```python
from build123d import *

# Parameters (mm, degrees)
F2_T     = -12.7
F3_R     = 76.2
F4_DEPTH = 781.3280539866
F6_DEPTH = 254
F7_COUNT = 24


with BuildPart() as f1:
    # F0 (on Front) → F1 (revolve)
    with BuildSketch(Plane.XZ):
        Polygon((-673.1, 0), (0, 0), (0, 781.3270539866), (-127, 781.3270539866), (-127, 400.3270539866), (-673.1, 254), align=None)
    revolve(axis=Axis((0, 0, 573.1903910637), (0, 0, 1)))

    # F2
    f2_openings = [f1.faces().sort_by_distance(p)[0] for p in [
        (0, 0, 0),
    ]]
    offset(amount=F2_T, openings=f2_openings, kind=Kind.INTERSECTION)

    # F3 (on face) → F4 (cut, through all)
    with BuildSketch(Plane.XY.offset(781.3270539866)):
        Circle(F3_R)
    extrude(amount=-F4_DEPTH, mode=Mode.SUBTRACT)

    # F5 (on face) → F6 (join)
    with BuildSketch(Plane(origin=(0, 0, 0), x_dir=(1, 0, 0), z_dir=(0, 0, -1))):
        with BuildLine():
            ThreePointArc((-644.4710936979, 194.2179687564), (-627.9881276024, 242.2695226199), (-607.9281554401, 288.9411148024))
            ThreePointArc((-607.9281554401, 288.9411148024), (-675.3834579875, 260.5540148931), (-644.4710936979, 194.2179687564))
        make_face()
    extrude(amount=-F6_DEPTH)

    # F7: F1 ×24 about axis
    f7_axis = Axis((0, 0, 768.6270539866), (0, 0, 1))


with BuildPart() as f1_1:
    add(f1.part)
    for i in range(1, F7_COUNT):
        add(f1.part.rotate(f7_axis, i * 360 / F7_COUNT))


solid = f1_1.part
```
Can you work these out from the model? Positions are in its coordinate system, mm. A direction names the side the tool comes from. Coordinates: 2 decimals unless noted, no trailing zeros. Loops run counter-clockwise (first coordinate to the right, second up) from the corner with the lowest first, then second, coordinate; pieces in that order, holes last. Notation, with made-up numbers: M -2.75,23 L 27.25,23 A18 ccw 27.25,51 Z; hole C -19.5,-23 d3. An arc over 180 degrees is marked long. Put each result on its own line as item: value. Start each with the question number.
(1) Will these pins go through, and if not, where does the flat tip stop? pin 1 Ø5 at (x, z) = (-377.5, 250) entering from +Y; pin 2 Ø8 at (x, y) = (572.5, -89.5) entering from -Z; pin 3 Ø4 at (y, z) = (-297.5, 101) entering from +X.
(2) Imagine slicing it at A-A on y = 0. List the corners of the cut face in (x, z) for me, and give its area (3 significant figures).
(3) We'd pull the mould along X, two halves only. Please class faces 4 (the face through (-244, 644, 254)), 5 (the face through (-351.178, -574.228, 125.222)): +X half, -X half, draft (parallel to the pull), parting line (faces both ways), or undercut.
(4) Imagine slicing it at C-C on z = 719. List the corners of the cut face in (x, y) for me.
(5) I need wall thicknesses on probe 1 along X at (y, z) = (0, 177); probe 2 along Y at (x, z) = (0, 776). Which ranges of each line are inside material? Lowest first, please.
(6) Which directions (+Z, -Z, +X, -X, +Y, -Y) give clear straight access to the entire face, cutting with the end or side of a thin tool? Please do faces 1 (the face through (628, -283, 254)), 2 (the face through (-463.77, 487.833, 125.222)), 3 (the face through (-644, -244, 254)).
Worked answers:
1. pin 1: stops at y = 591.91
1. pin 2: stops at z = 264.87
1. pin 3: stops at x = 660.78
2. outline: M -673.1,0 L -660.4,0 L -660.4,244.25 L -114.3,390.58 L -114.3,768.63 L -76.2,768.63 L -76.2,781.33 L -127,781.33 L -127,400.33 L -673.1,254 Z; M 76.2,768.63 L 114.3,768.63 L 114.3,390.58 L 660.4,244.25 L 660.4,0 L 673.1,0 L 673.1,254 L 127,400.33 L 127,781.33 L 76.2,781.33 Z
2. area: 31,500 mm2
3. face 4: draft
3. face 5: undercut
4. outline: C 0,0 d254; hole C 0,0 d228.6
5. probe 1: x = -673.1 to -660.4, 660.4 to 673.1
5. probe 2: y = -127 to -76.2, 76.2 to 127
6. face 1: +Z, +X, -Y
6. face 2: +Z, -Z
6. face 3: +Z, -X, -Y
